Design review of the part built by this model. Coordinates are the model's own, in mm. A direction names the side the tool comes from. Coordinates: 2 decimals unless noted, no trailing zeros. Loops run counter-clockwise (first coordinate to the right, second up) from the corner with the lowest first, then second, coordinate; pieces in that order, holes last. Notation, with made-up numbers: (28, 79.25) - (54, 79.25) arc R19 ccw to (54, 96.25) - close; hole circle Ø4 at (63, 68.5). An arc over 180 degrees is marked (long way). Use one line per item in the form item = value. Start each with the question number.
(1) Add section B-B (x = 32.5). State the section outline as (y, z) points, plus the area to 3 significant figures.
(2) Tool access review of faces 1 (the face through (15, 12, 0)), 2 (the face through (36.39, 18.46, 2.89)), 3 (the face through (-7, 4.5, 4)), 4 (the face through (41.323, 13.5, 3.8)), 5 (the face through (29, 12.3, 4)): name each direction out of +Z, -Z, +X, -X, +Y, -Y from which nothing blocks a thin tool from reaching the whole face with its end or side.
(3) The part is to be moulded in two halves that separate along Z. For faces 6 (the face through (-10.218, 2, 4)), 7 (the face through (31.323, 16, 4)), 8 (the face through (15, 12, 7.7)), say which applies: pulls with the +Z half, pulls with the -Z half, needs draft (parallel to the pull), parting line crosses it, or undercut.
(4) Add section A-A (z = 3.85). State the section outline as (x, y) points.
(5) Add section D-D (y = 16.15). State the section outline as (x, z) points, plus the area to 3 significant figures.
(6) Clearance check with a flat-ended pin moving along its axis: pin 1 Ø4.5 at (x, z) = (-6, 4.5) entering from +Y. State where the tip first meets the part, or that it passes through.
(7) For L1, parallel to Z at x = 35, y = 16.15; L2, parallel to Y at x = 29, z = 4.25; L3, parallel to X at y = 11.5, z = 5.25, list the stretches that pass through material, from the lowest coordinate up.
(8) Add section C-C (y = 2.75). State the section outline as (x, z) points, plus the area to 3 significant figures.
```python
from build123d import *

# Parameters (mm, degrees)
EXTRUDE_408_DEPTH      = 7.7
FILLET_1_R             = 3
SKETCH_4_R             = 2.5
CUT_EXTRUDE_703_DEPTH  = 10
SKETCH_5_R             = 1
CUT_EXTRUDE_1066_DEPTH = 47.549452316
FILLET_3_R             = 0.5


with BuildPart() as part:
    # 草图1 → Extrude 408 (new body)
    with BuildSketch(Plane.XY):
        Polygon((0, 0), (16.322651306, 12.3), (41.322651306, 12.3), (41.322651306, 20), (16.322651306, 20), (-4.246543429, 4.5), (-10.218245126, 4.5), (-10.218245126, 0), align=None)
    extrude(amount=EXTRUDE_408_DEPTH)

    # 圆角1
    fillet_1_edges = [part.edges().sort_by_distance(p)[0] for p in [
        (16.322651306, 20, 3.85),
    ]]
    fillet(fillet_1_edges, radius=FILLET_1_R)

    # 草图4 → Cut-Extrude 703 (cut)
    with BuildSketch(Plane(origin=(41.322651306, 0, 0), x_dir=(0, 0, -1), z_dir=(1, 0, 0))):
        with Locations(Location((-3.85, 16.15, 0), (0, 0, 90))):
            Circle(SKETCH_4_R)
    extrude(amount=-CUT_EXTRUDE_703_DEPTH, mode=Mode.SUBTRACT)

    # 草图5 → Cut-Extrude 1066 (cut, through all)
    with BuildSketch(Plane.XZ):
        with Locations((-5.409122563, 3.85)):
            Circle(SKETCH_5_R)
    extrude(amount=-CUT_EXTRUDE_1066_DEPTH, mode=Mode.SUBTRACT)

    # 圆角3
    fillet_3_edges = [part.edges().sort_by_distance(p)[0] for p in [
        (-10.218245126, 4.5, 3.85),
    ]]
    fillet(fillet_3_edges, radius=FILLET_3_R)


solid = part.part
```
Computed values:
q1.outline = (12.3, 0) - (20, 0) - (20, 7.7) - (12.3, 7.7) - close; hole circle Ø5 at (16.15, 3.85)
q1.area = 39.7 mm^2
q2.face_1 = -Z, +X, -X, +Y, -Y
q2.face_2 = +X
q2.face_3 = +Z, -Z, -X, +Y
q2.face_4 = +Z, -Z, +X, +Y, -Y
q2.face_5 = +Z, -Z, +X, -Y
q3.face_6 = needs draft
q3.face_7 = undercut
q3.face_8 = pulls with the +Z half
q4.outline = (-10.22, 0) - (-6.41, 0) - (-6.41, 4.5) - (-9.72, 4.5) arc R0.5 ccw to (-10.22, 4) - close; (-4.41, 0) - (0, 0) - (16.32, 12.3) - (41.32, 12.3) - (41.32, 13.65) - (31.32, 13.65) - (31.32, 18.65) - (41.32, 18.65) - (41.32, 20) - (17.33, 20) arc R3 ccw to (15.52, 19.4) - (-4.25, 4.5) - (-4.41, 4.5) - close
q5.outline = (11.21, 0) - (41.32, 0) - (41.32, 1.35) - (31.32, 1.35) - (31.32, 6.35) - (41.32, 6.35) - (41.32, 7.7) - (11.21, 7.7) - close
q5.area = 182 mm^2
q6.pin_1 = 4.87
q7.L1 = 0 to 1.35, 6.35 to 7.7
q7.L2 = 12.3 to 20
q7.L3 = 5.04 to 15.26
q8.outline = (-10.22, 0) - (3.65, 0) - (3.65, 7.7) - (-10.22, 7.7) - close; hole circle Ø2 at (-5.41, 3.85)
q8.area = 104 mm^2
